Verification items for the finished model (mm, model axes). A direction names the side the tool comes from. Give positions to 0.01 mm unless a question says otherwise; leave off trailing zeros. Write each loop counter-clockwise with the first axis right and the second up, starting at its lowest first coordinate (ties: lowest second). Pieces come first, ordered by that corner, then holes. Notation, with made-up numbers: (34, 83.25) -> (53, 83.25) arc R6 ccw to (53, 92.25) -> close; hole circle Ø3 at (40, 87). An arc over 180 degrees is marked (long way). Use CSV: the item, a comma, the result in double quotes. Start each with the question number.
```python
from build123d import *

# Parameters (mm, degrees)
SALIENTE_EXTRUIR1_DEPTH = 4
CROQUIS5_R              = 2.6
CORTAR_EXTRUIR3_DEPTH   = 5
CORTAR_EXTRUIR4_DEPTH   = 5
CROQUIS10_R             = 1.5
CORTAR_EXTRUIR5_DEPTH   = 5
CROQUIS4_W              = 6.15
CROQUIS4_H              = 53
CORTAR_EXTRUIR6_DEPTH   = 0.1


with BuildPart() as part:
    # Croquis1 → Saliente-Extruir1 (new body)
    with BuildSketch(Plane(origin=(0, 0, 0), x_dir=(1, 0, 0), z_dir=(0, 1, 0))):
        with BuildLine():
            Line((-5.775, -25), (5.775, -25))
            ThreePointArc((5.775, -25), (9.310533906, -23.535533906), (10.775, -20))
            Line((10.775, -20), (10.775, -14))
            Line((10.775, -14), (15.775, -14))
            Line((15.775, -14), (15.775, -8))
            Line((15.775, -8), (10.775, -8))
            Line((10.775, -8), (10.775, -1.55))
            Line((10.775, -1.55), (8.725, -1.55))
            Line((8.725, -1.55), (8.725, -2.8))
            Line((8.725, -2.8), (5.825, -2.8))
            Line((5.825, -2.8), (5.825, -1.55))
            Line((5.825, -1.55), (3.775, -1.55))
            Line((3.775, -1.55), (3.775, 1.55))
            Line((3.775, 1.55), (5.825, 1.55))
            Line((5.825, 1.55), (5.825, 2.8))
            Line((5.825, 2.8), (8.725, 2.8))
            Line((8.725, 2.8), (8.725, 1.55))
            Line((8.725, 1.55), (10.775, 1.55))
            Line((10.775, 1.55), (10.775, 8))
            Line((10.775, 8), (15.775, 8))
            Line((15.775, 8), (15.775, 14))
            Line((15.775, 14), (10.775, 14))
            Line((10.775, 14), (10.775, 20))
            ThreePointArc((10.775, 20), (9.310533906, 23.535533906), (5.775, 25))
            Line((5.775, 25), (-5.775, 25))
            ThreePointArc((-5.775, 25), (-9.310533906, 23.535533906), (-10.775, 20))
            Line((-10.775, 20), (-10.775, -20))
            ThreePointArc((-10.775, -20), (-9.310533906, -23.535533906), (-5.775, -25))
        make_face()
    extrude(amount=SALIENTE_EXTRUIR1_DEPTH)

    # Croquis5 → Cortar-Extruir3 (cut, through all)
    with BuildSketch(Plane(origin=(0, 4, 0), x_dir=(1, 0, 0), z_dir=(0, 1, 0))):
        with Locations((-6.775, 11.5)):
            Circle(CROQUIS5_R)
        with Locations((5.225, 11.5)):
            Circle(CROQUIS5_R)
        with Locations((5.225, -11.5)):
            Circle(CROQUIS5_R)
        with Locations((-6.775, -11.5)):
            Circle(CROQUIS5_R)
    extrude(amount=-CORTAR_EXTRUIR3_DEPTH, mode=Mode.SUBTRACT)

    # Croquis7 → Cortar-Extruir4 (cut, through all)
    with BuildSketch(Plane(origin=(0, 4, 0), x_dir=(1, 0, 0), z_dir=(0, 1, 0))):
        with BuildLine():
            Line((9.152341989, 1.55), (10.775, 1.55))
            Line((10.775, 1.55), (10.775, -1.55))
            Line((10.775, -1.55), (9.152341989, -1.55))
            ThreePointArc((9.152341989, -1.55), (8.650478098, -2.869619136), (7.275, -3.187930349))
            ThreePointArc((7.275, -3.187930349), (6.030747615, -2.971867524), (5.392475162, -1.882163243))
            ThreePointArc((5.392475162, -1.882163243), (3.80076038, -1.575149398), (3.41772275, 0))
            ThreePointArc((3.41772275, 0), (3.80076038, 1.575149398), (5.392475162, 1.882163243))
            ThreePointArc((5.392475162, 1.882163243), (6.030747615, 2.971867524), (7.275, 3.187930349))
            ThreePointArc((7.275, 3.187930349), (8.650478098, 2.869619136), (9.152341989, 1.55))
        make_face()
    extrude(amount=-CORTAR_EXTRUIR4_DEPTH, mode=Mode.SUBTRACT)

    # Croquis10 → Cortar-Extruir5 (cut, through all)
    with BuildSketch(Plane(origin=(0, 4, 0), x_dir=(1, 0, 0), z_dir=(0, 1, 0))):
        with Locations((11.835660172, 15.060660172)):
            Circle(CROQUIS10_R)
        with Locations((11.835660172, 6.939339828)):
            Circle(CROQUIS10_R)
        with Locations((11.835660172, -15.060660172)):
            Circle(CROQUIS10_R)
        with Locations((11.835660172, -6.939339828)):
            Circle(CROQUIS10_R)
    extrude(amount=-CORTAR_EXTRUIR5_DEPTH, mode=Mode.SUBTRACT)

    # Croquis4 → Cortar-Extruir6 (cut)
    with BuildSketch(Plane(origin=(0, 0, 0), x_dir=(1, 0, 0), z_dir=(0, 1, 0))):
        with Locations((-0.775, 0)):
            Rectangle(CROQUIS4_W, CROQUIS4_H)
    extrude(amount=CORTAR_EXTRUIR6_DEPTH, mode=Mode.SUBTRACT)


solid = part.part
```
(1) Section check A-A on z = 11.5. Record the cut outline in (x, y) (3 decimals), then the cut area to 3 significant figures.
(2) Set-up check for faces 1 (the face through (14, 2, -14)), 2 (the face through (14, 2, 8)), 3 (the face through (10.775, 2, 18)): record each of +Z, -Z, +X, -X, +Y, -Y from which the full face is reachable in a straight line by a thin tool's end or side.
(3) Thickness scan on line 1 (X direction, y = 3, z = 11.5) (3 decimals); line 2 (Z direction, x = 13.25, y = 1.8); line 3 (X direction, y = 3.25, z = 10) (3 decimals). Record the ranges inside material, lowest first. Write a range as from..to.
(4) Section check D-D on z = -4.5. Record the cut outline in (x, y) (3 decimals), then the cut area to 3 significant figures.
(5) Section check B-B on y = 1.75. Give the number of separate pieces and of enclosed holes in the cut face, then the cut area to 3 significant figures.
(6) Draft check along X on faces 4 (the face through (-10.775, 2, 0)), 5 (the face through (9.349, 1.972, -23.496)), 6 (the face through (-7.339, 2.028, 14.038)). Enter one of: released by +X, released by -X, zero draft, split by the parting line, or undercut.
(7) Section check C-C on x = -7. Record the cut outline in (y, z).
(8) Go/stop test with flat-tipped pins: pin 1 (1.4 mm diameter, centred on x = 14.5, y = 3, fed in from +Z); pin 2 (2 mm diameter, centred on y = 1, z = 4, fed in from +X) (3 decimals); pin 3 (1.8 mm diameter, centred on x = 9.5, y = 2.5, fed in from -Z). Record where each tip stops, or that it passes through.
Data:
1,outline,"(-10.775, 0) -> (-9.375, 0) -> (-9.375, 4) -> (-10.775, 4) -> close; (-4.175, 0) -> (-3.85, 0) -> (-3.85, 0.1) -> (2.3, 0.1) -> (2.3, 0) -> (2.625, 0) -> (2.625, 4) -> (-4.175, 4) -> close; (7.825, 0) -> (15.775, 0) -> (15.775, 4) -> (7.825, 4) -> close"
1,area,"64.0 mm2"
2,face 1,"-Z, +X, +Y, -Y"
2,face 2,"+X, +Y, -Y"
2,face 3,"+Z, +X, +Y, -Y"
3,line 1,"x = -10.775..-9.375, -4.175..2.625, 7.825..15.775"
3,line 2,"z = -14..-8, 8..14"
3,line 3,"x = -10.775..-8.899, -4.651..3.101, 7.349..15.775"
4,outline,"(-10.775, 0) -> (-3.85, 0) -> (-3.85, 0.1) -> (2.3, 0.1) -> (2.3, 0) -> (10.775, 0) -> (10.775, 4) -> (-10.775, 4) -> close"
4,area,"85.6 mm2"
5,separate pieces,"1"
5,enclosed holes,"4"
5,area,"991 mm2"
6,face 4,"released by -X"
6,face 5,"released by +X"
6,face 6,"undercut"
7,outline,"(0, -24.85) -> (4, -24.85) -> (4, -14.09) -> (0, -14.09) -> close; (0, -8.91) -> (4, -8.91) -> (4, 8.91) -> (0, 8.91) -> close; (0, 14.09) -> (4, 14.09) -> (4, 24.85) -> (0, 24.85) -> close"
8,pin 1,"stops at z = 14"
8,pin 2,"stops at x = 10.775"
8,pin 3,"stops at z = -24.13"
